Answer from the drawing. Dimensions are ordinates in mm from the lowest x, y and z of the part. A direction names the side the tool comes from. Give positions to 0.01 mm unless a question says otherwise; leave off trailing zeros. Write each loop counter-clockwise with the first axis right and the second up, starting at its lowest first coordinate (ties: lowest second). Pieces come first, ordered by that corner, then holes. Notation, with made-up numbers: M 31.25,3 L 50.25,3 A19 cw 50.25,12 Z; hole C 2.5,7.25 d10. An arc over 180 degrees is marked long. Answer as a JSON object with one key per item and string values.
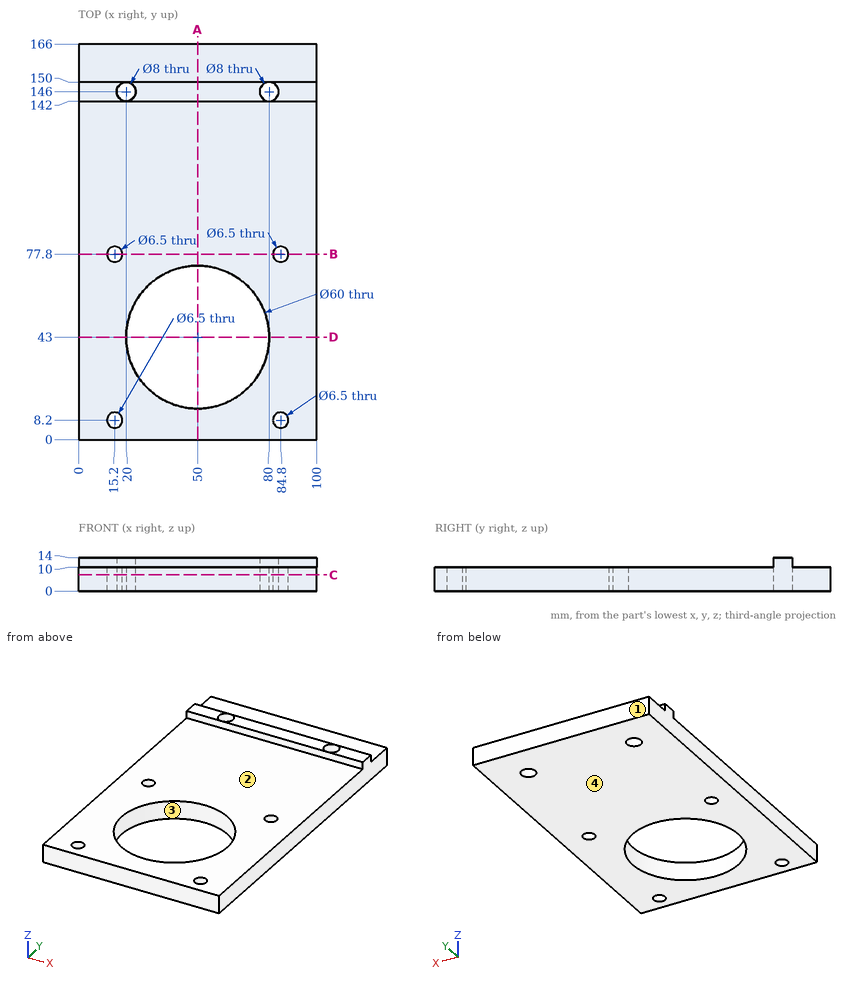
1. A cutting plane is placed at D-D, the plane y = 43. Give the vertices of the cut face in (x, z).
Verdict:
{"outline": "M 0,0 L 20,0 L 20,10 L 0,10 Z; M 80,0 L 100,0 L 100,10 L 80,10 Z"}
2. A cutting plane is placed at C-C, the plane z = 6.75. Give the vertices of the cut face in (x, y), plus the area to 3 significant figures.
Verdict:
{"outline": "M 0,0 L 100,0 L 100,166 L 0,166 Z; hole C 15.2,8.2 d6.5; hole C 15.2,77.8 d6.5; hole C 20,146 d8; hole C 50,43 d60; hole C 80,146 d8; hole C 84.8,8.2 d6.5; hole C 84.8,77.8 d6.5", "area": "13,500 mm2"}
3. A cutting plane is placed at B-B, the plane y = 77.8. Give the vertices of the cut face in (x, z), plus the area to 3 significant figures.
Verdict:
{"outline": "M 0,0 L 11.95,0 L 11.95,10 L 0,10 Z; M 18.45,0 L 81.55,0 L 81.55,10 L 18.45,10 Z; M 88.05,0 L 100,0 L 100,10 L 88.05,10 Z", "area": "870 mm2"}
4. A cutting plane is placed at A-A, the plane x = 50. Give the vertices of the cut face in (y, z), plus the area to 3 significant figures.
Verdict:
{"outline": "M 0,0 L 13,0 L 13,10 L 0,10 Z; M 73,0 L 166,0 L 166,10 L 150,10 L 150,14 L 142,14 L 142,10 L 73,10 Z", "area": "1,090 mm2"}
5. Consider line 1 along Y through (x, z) = (15.2, 4); line 2 along X through (y, z) = (146, 9.75); line 3 along X through (y, z) = (144.5, 4). Determine where each line is inside the solid, lowest interval first.
Verdict:
{"line 1": "y = 0 to 4.95, 11.45 to 74.55, 81.05 to 166", "line 2": "x = 0 to 16, 24 to 76, 84 to 100", "line 3": "x = 0 to 16.29, 23.71 to 76.29, 83.71 to 100"}
6. For the marked faces 1 and 2, determine the directions among +Z, -Z, +X, -X, +Y, -Y from which every point of the face is accessible in a straight line to the end or side of a thin tool.
Verdict:
{"face 1": "+Z, -Z, +X, -X, +Y", "face 2": "+Z, +X, -X, -Y"}
7. The mould has two halves that part along X. Classify the marked faces 3 and 4: released by +X, released by -X, zero draft, split by the parting line, or undercut.
Verdict:
{"face 3": "undercut", "face 4": "zero draft"}
8. A flat-ended cylindrical pin translates along its axis: pin 1 (6 mm diameter, centred on x = 84.8, y = 8.2, fed in from -Z). Find the tip coordinate at first contact, or state that the pin passes through.
Verdict:
{"pin 1": "passes through"}
